Here's the drawing with two shaded views (mm, measured from the low corner). I have some questions. Give positions to 0.01 mm unless a question says otherwise; leave off trailing zeros. Loops run counter-clockwise (first coordinate to the right, second up) from the corner with the lowest first, then second, coordinate; pieces in that order, holes last.
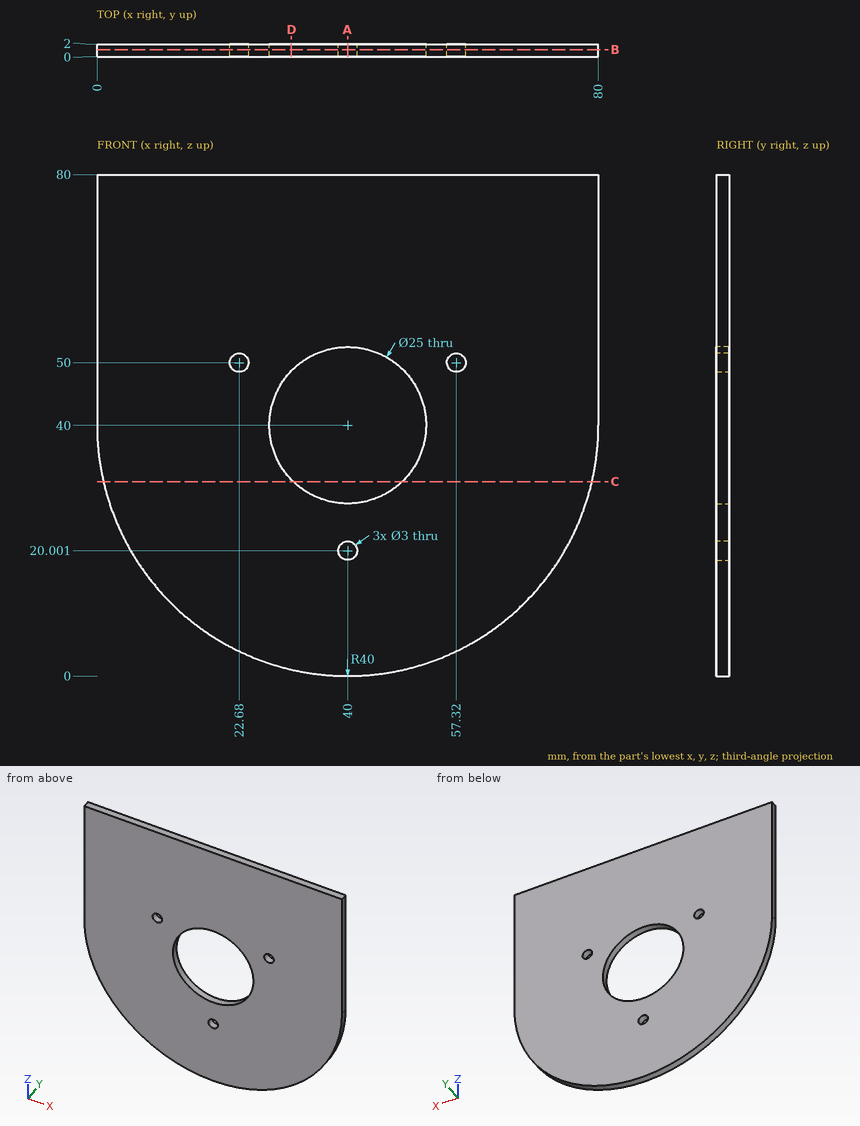
(1) Suppose I cut it at B-B on y = 1.1. List the corners of the cut face in (x, z) for me, plus the area to 3 significant figures.
Returned:
outline: (0, 40) arc R40 ccw to (80, 40) - (80, 80) - (0, 80) - close; hole circle Ø3 at (22.68, 50); hole circle Ø25 at (40, 40); hole circle Ø3 at (40, 20); hole circle Ø3 at (57.32, 50)
area: 5,200 mm2
(2) Please list where these lines run through material, in increasing order: probe 1 along X at (y, z) = (1.2, 40); probe 2 along X at (y, z) = (0.5, 36); probe 3 along Z at (x, y) = (56.5, 1.1) (1 decimal).
Returned:
probe 1: x = 0 to 27.5, 52.5 to 80
probe 2: x = 0.2 to 28.16, 51.84 to 79.8
probe 3: z = 3.6 to 48.7, 51.3 to 80
(3) Suppose I cut it at A-A on x = 40. List the corners of the cut face in (y, z) for me, plus the area to 3 significant figures.
Returned:
outline: (0, 0) - (2, 0) - (2, 18.5) - (0, 18.5) - close; (0, 21.5) - (2, 21.5) - (2, 27.5) - (0, 27.5) - close; (0, 52.5) - (2, 52.5) - (2, 80) - (0, 80) - close
area: 104 mm2
(4) Suppose I cut it at C-C on z = 31. List the corners of the cut face in (x, y) for me (1 decimal).
Returned:
outline: (1, 0) - (31.3, 0) - (31.3, 2) - (1, 2) - close; (48.7, 0) - (79, 0) - (79, 2) - (48.7, 2) - close
(5) Suppose I cut it at D-D on x = 31. List the corners of the cut face in (y, z) for me (1 decimal), plus the area to 3 significant figures.
Returned:
outline: (0, 1) - (2, 1) - (2, 31.3) - (0, 31.3) - close; (0, 48.7) - (2, 48.7) - (2, 80) - (0, 80) - close
area: 123 mm2
